Source: three-view drawing plus pictorial views. Frame: mm from the lowest corner of the part. Give positions to 0.01 mm unless a question says otherwise; leave off trailing zeros. Order: outer loops, then holes, each group sorted by start corner. A loop starts at its lowest first (then second) coordinate and runs counter-clockwise, first axis right, second up. Notation, with made-up numbers: (29, 15) - (39, 15) arc R23 cw to (39, 41) - close; hole circle Ø2 at (-26, 4). An arc over 180 degrees is marked (long way). Use one line per item in the form item = value.
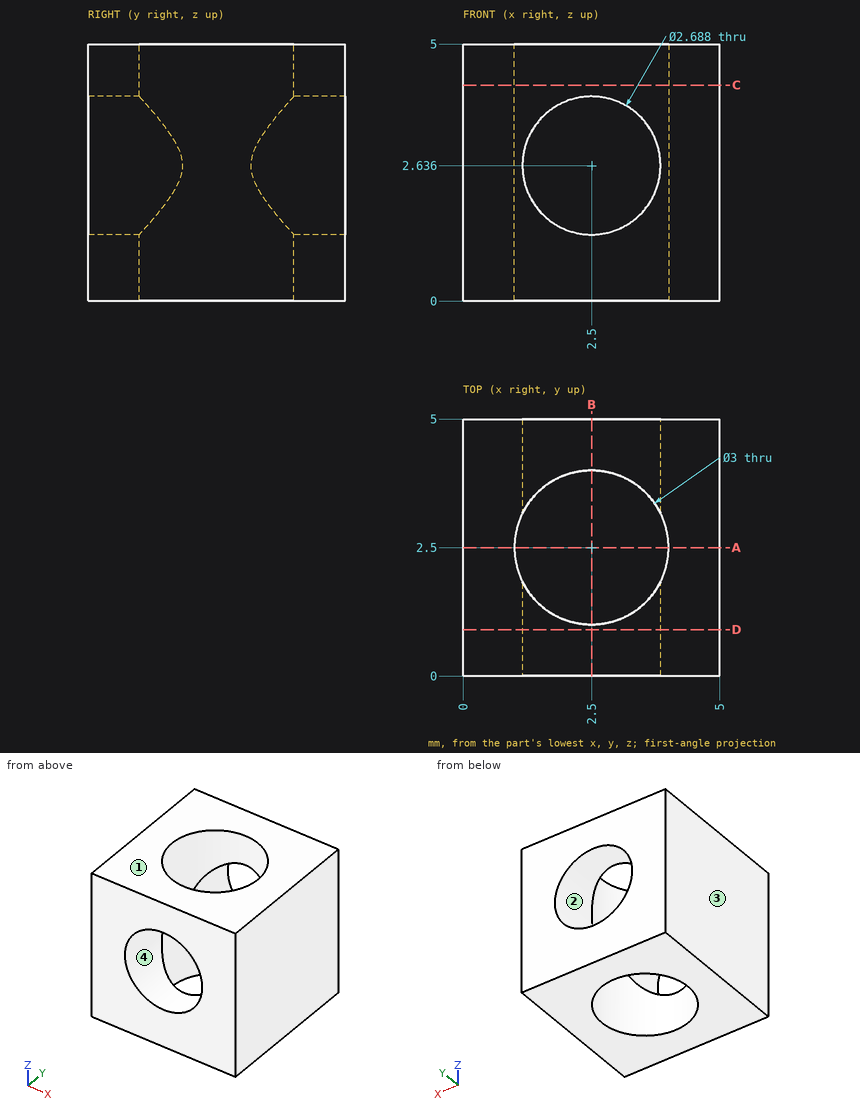
(1) Cut plane A-A on y = 2.5. Output: boundary loops of the cut face in (x, z), plus the area to 3 significant figures.
Computed values:
outline = (0, 0) - (1, 0) - (1, 5) - (0, 5) - close; (4, 0) - (5, 0) - (5, 5) - (4, 5) - close
area = 10.0 mm²
(2) Cut plane D-D on y = 0.9. Output: boundary loops of the cut face in (x, z) (1 decimal), plus the area to 3 significant figures.
Computed values:
outline = (0, 0) - (5, 0) - (5, 5) - (0, 5) - close; hole circle Ø2.7 at (2.5, 2.6)
area = 19.3 mm²
(3) Ray query, line 1 along Z through (x, y) = (2.5, 0.95); line 2 along Z through (x, y) = (2.15, 4.6); line 3 along X through (y, z) = (1.8, 2.8) (1 decimal). Return the intervals inside material, ascending.
Computed values:
line_1 = 0 to 1.29, 3.98 to 5
line_2 = 0 to 1.34, 3.93 to 5
line_3 = 0 to 1.2, 3.8 to 5
(4) Cut plane C-C on z = 4.2. Output: boundary loops of the cut face in (x, y).
Computed values:
outline = (0, 0) - (5, 0) - (5, 5) - (0, 5) - close; hole circle Ø3 at (2.5, 2.5)
(5) Pull-direction query (X, two-part tool) for the marked faces 1, 2, 3 and 4; classes: released by +X, released by -X, zero draft, split by the parting line, or undercut.
Computed values:
face_1 = zero draft
face_2 = undercut
face_3 = released by -X
face_4 = undercut
(6) Cut plane B-B on x = 2.5. Output: boundary loops of the cut face in (y, z).
Computed values:
outline = (0, 0) - (1, 0) - (1, 1.29) - (0, 1.29) - close; (0, 3.98) - (1, 3.98) - (1, 5) - (0, 5) - close; (4, 0) - (5, 0) - (5, 1.29) - (4, 1.29) - close; (4, 3.98) - (5, 3.98) - (5, 5) - (4, 5) - close
